from build123d import *

# Parameters (mm, degrees)
SKETCH_2_W          = 180
SKETCH_2_H          = 180
EXTRUDE_1_DEPTH     = 5
EXTRUDE_1_2_DEPTH   = 115
EXTRUDE_2_DEPTH     = 2
CUT_EXTRUDE_1_DEPTH = 140.5
SKETCH_6_R          = 6.5
CUT_EXTRUDE_2_DEPTH = 6
FILLET_1_R          = 10
CUT_EXTRUDE_3_REACH = 141


with BuildPart() as part:
    # Эскиз2 → Extrude 1 (new body)
    with BuildSketch(Plane(origin=(0, 0, 0), x_dir=(1, 0, 0), z_dir=(0, 1, 0))):
        Rectangle(SKETCH_2_W, SKETCH_2_H)
    extrude(amount=EXTRUDE_1_DEPTH)

    # Эскиз3 → Extrude 1 2 (add)
    with BuildSketch(Plane(origin=(0, 5, 0), x_dir=(1, 0, 0), z_dir=(0, 1, 0))):
        with BuildLine():
            Line((-45.5, -45), (-45.5, 44))
            ThreePointArc((-45.5, 44), (-45.207106781, 44.707106781), (-44.5, 45))
            Line((-44.5, 45), (44.5, 45))
            ThreePointArc((44.5, 45), (45.207106781, 44.707106781), (45.5, 44))
            Line((45.5, 44), (45.5, -45))
            Line((45.5, -45), (49.5, -45))
            Line((49.5, -45), (49.5, 44))
            ThreePointArc((49.5, 44), (48.035533906, 47.535533906), (44.5, 49))
            Line((44.5, 49), (-44.5, 49))
            ThreePointArc((-44.5, 49), (-48.035533906, 47.535533906), (-49.5, 44))
            Line((-49.5, 44), (-49.5, -45))
            Line((-49.5, -45), (-45.5, -45))
        make_face()
    extrude(amount=EXTRUDE_1_2_DEPTH)

    # Эскиз4 → Бобышка-Вытянуть2 (add, symmetric)
    with BuildSketch(Plane(origin=(0, 0, 0), x_dir=(0, 0, -1), z_dir=(1, 0, 0))):
        Polygon((49, 67.353829072), (85, 5), (49, 5), align=None)
    extrude(amount=EXTRUDE_2_DEPTH, both=True)

    # Эскиз5 → Вырез-Вытянуть1 (cut, through all)
    with BuildSketch(Plane(origin=(49.5, 0, 0), x_dir=(0, 0, -1), z_dir=(1, 0, 0))):
        with BuildLine():
            Line((-17.5, 108), (-17.5, 96))
            ThreePointArc((-17.5, 96), (-22.5, 91), (-27.5, 96))
            Line((-27.5, 96), (-27.5, 108))
            ThreePointArc((-27.5, 108), (-22.5, 113), (-17.5, 108))
        make_face()
        with BuildLine():
            Line((-17.5, 29), (-17.5, 17))
            ThreePointArc((-17.5, 17), (-22.5, 12), (-27.5, 17))
            Line((-27.5, 17), (-27.5, 29))
            ThreePointArc((-27.5, 29), (-22.5, 34), (-17.5, 29))
        make_face()
        with BuildLine():
            Line((17.5, 108), (17.5, 96))
            ThreePointArc((17.5, 96), (22.5, 91), (27.5, 96))
            Line((27.5, 96), (27.5, 108))
            ThreePointArc((27.5, 108), (22.5, 113), (17.5, 108))
        make_face()
        with BuildLine():
            Line((17.5, 29), (17.5, 17))
            ThreePointArc((17.5, 17), (22.5, 12), (27.5, 17))
            Line((27.5, 17), (27.5, 29))
            ThreePointArc((27.5, 29), (22.5, 34), (17.5, 29))
        make_face()
    extrude(amount=-CUT_EXTRUDE_1_DEPTH, mode=Mode.SUBTRACT)

    # Эскиз6 → Вырез-Вытянуть2 (cut, through all)
    with BuildSketch(Plane(origin=(0, 5, 0), x_dir=(1, 0, 0), z_dir=(0, 1, 0))):
        with Locations(Location((-75, 75, 0), (0, 0, 270))):  # turned: the seam where the file's is
            Circle(SKETCH_6_R)
        with Locations(Location((-75, -75, 0), (0, 0, 270))):  # turned: the seam where the file's is
            Circle(SKETCH_6_R)
        with Locations(Location((75, 75, 0), (0, 0, 270))):  # turned: the seam where the file's is
            Circle(SKETCH_6_R)
        with Locations(Location((75, -75, 0), (0, 0, 270))):  # turned: the seam where the file's is
            Circle(SKETCH_6_R)
    extrude(amount=-CUT_EXTRUDE_2_DEPTH, mode=Mode.SUBTRACT)

    # Скругление1
    fillet_1_edges = [part.edges().sort_by_distance(p)[0] for p in [
        (90, 2.5, 90),
        (-90, 2.5, 90),
        (-90, 2.5, -90),
        (90, 2.5, -90),
    ]]
    fillet(fillet_1_edges, radius=FILLET_1_R)

    # Эскиз8 → Вырез-Вытянуть3 (cut, up to next)
    with BuildSketch(Plane(origin=(0, 0, -49), x_dir=(-1, 0, 0), z_dir=(0, 0, -1)), mode=Mode.PRIVATE) as cut_extrude_3_sk1:
        with BuildLine():
            Line((-17.5, 108), (-17.5, 96))
            ThreePointArc((-17.5, 96), (-22.5, 91), (-27.5, 96))
            Line((-27.5, 96), (-27.5, 108))
            ThreePointArc((-27.5, 108), (-22.5, 113), (-17.5, 108))
        make_face()
    cut_extrude_3_tool1 = extrude(cut_extrude_3_sk1.sketch, amount=-CUT_EXTRUDE_3_REACH, mode=Mode.PRIVATE) & part.part
    add(cut_extrude_3_tool1.solids().sort_by_distance((22.5, 102, -49))[0], mode=Mode.SUBTRACT)
    # Эскиз8 → Вырез-Вытянуть3 (cut, up to next)
    with BuildSketch(Plane(origin=(0, 0, -49), x_dir=(-1, 0, 0), z_dir=(0, 0, -1)), mode=Mode.PRIVATE) as cut_extrude_3_sk2:
        with BuildLine():
            Line((-17.5, 29), (-17.5, 17))
            ThreePointArc((-17.5, 17), (-22.5, 12), (-27.5, 17))
            Line((-27.5, 17), (-27.5, 29))
            ThreePointArc((-27.5, 29), (-22.5, 34), (-17.5, 29))
        make_face()
    cut_extrude_3_tool2 = extrude(cut_extrude_3_sk2.sketch, amount=-CUT_EXTRUDE_3_REACH, mode=Mode.PRIVATE) & part.part
    add(cut_extrude_3_tool2.solids().sort_by_distance((22.5, 23, -49))[0], mode=Mode.SUBTRACT)
    # Эскиз8 → Вырез-Вытянуть3 (cut, up to next)
    with BuildSketch(Plane(origin=(0, 0, -49), x_dir=(-1, 0, 0), z_dir=(0, 0, -1)), mode=Mode.PRIVATE) as cut_extrude_3_sk3:
        with BuildLine():
            Line((17.5, 108), (17.5, 96))
            ThreePointArc((17.5, 96), (22.5, 91), (27.5, 96))
            Line((27.5, 96), (27.5, 108))
            ThreePointArc((27.5, 108), (22.5, 113), (17.5, 108))
        make_face()
    cut_extrude_3_tool3 = extrude(cut_extrude_3_sk3.sketch, amount=-CUT_EXTRUDE_3_REACH, mode=Mode.PRIVATE) & part.part
    add(cut_extrude_3_tool3.solids().sort_by_distance((-22.5, 102, -49))[0], mode=Mode.SUBTRACT)
    # Эскиз8 → Вырез-Вытянуть3 (cut, up to next)
    with BuildSketch(Plane(origin=(0, 0, -49), x_dir=(-1, 0, 0), z_dir=(0, 0, -1)), mode=Mode.PRIVATE) as cut_extrude_3_sk4:
        with BuildLine():
            Line((17.5, 29), (17.5, 17))
            ThreePointArc((17.5, 17), (22.5, 12), (27.5, 17))
            Line((27.5, 17), (27.5, 29))
            ThreePointArc((27.5, 29), (22.5, 34), (17.5, 29))
        make_face()
    cut_extrude_3_tool4 = extrude(cut_extrude_3_sk4.sketch, amount=-CUT_EXTRUDE_3_REACH, mode=Mode.PRIVATE) & part.part
    add(cut_extrude_3_tool4.solids().sort_by_distance((-22.5, 23, -49))[0], mode=Mode.SUBTRACT)


solid = part.part
Read the model definition and answer for the solid it produces. Units are mm, in the model's axes. A direction names the side the tool comes from. Give positions to 0.01 mm unless a question says otherwise; leave off trailing zeros. Write each loop counter-clockwise with the first axis right and the second up, starting at its lowest first coordinate (ties: lowest second). Pieces come first, ordered by that corner, then holes. Notation, with made-up numbers: (77.25, -17.5) - (84.25, -17.5) arc R16 cw to (84.25, 3.5) - close; hole circle Ø5 at (7, 21.5). An arc over 180 degrees is marked (long way). Answer in a Markdown table with one row per item. Add a question column.
Item 1: Section D-D, the plane y = 76.5 is taken. Write down the section's boundary in (x, z), and give its area (3 significant figures).
Item 2: Section B-B, the plane z = 75 is taken. Write down the section's boundary in (x, y), and give its area (3 significant figures).
Item 3: Flat-ended cylindrical pins translate along their axes: P1, Ø2, axis at x = -48, y = 23, coming from the +Z side; P2, Ø8, axis at x = -4, y = 100.5, coming from the +Z side; P3, Ø4.5, axis at y = 22.5, z = -47.5, coming from the -X side. Find the tip coordinate at first contact, or state that the pin passes through.
Item 4: Section C-C, the plane z = -22.5 is taken. Write down the section's boundary in (x, y).
Item 5: Find the intervals of material crossed by L1, parallel to X at y = 3.7, z = -75; L2, parallel to X at y = 81, z = 13; L3, parallel to Y at x = 63, z = -40.5, in increasing order.
Item 6: A tool of negligible diameter and unlimited length cuts with its end or side. For faces 4 (the face through (-9, 62, -49)), 5 (the face through (49.5, 62, 1)), 6 (the face through (-45.5, 62, 1)), from which of +Z, -Z, +X, -X, +Y, -Y can it reach the whole face along a straight path? Write none if from no direction.
Item 7: Determine the mould class of faces 1 (the face through (-87.15, 2.54, 86.99)), 2 (the face through (22.6, 34, -47)), 3 (the face through (47.5, 34, -22.6)) for opening direction X: pulls with the +X half, pulls with the -X half, needs draft (parallel to the pull), parting line crosses it, or undercut.
Item 8: Section A-A, the plane x = 75 is taken. Write down the section's boundary in (y, z), and give its area (3 significant figures).
Recorded:
| question | item | result |
|---|---|---|
| 1 | outline | (-49.5, -44) arc R5 ccw to (-44.5, -49) - (44.5, -49) arc R5 ccw to (49.5, -44) - (49.5, 45) - (45.5, 45) - (45.5, -44) arc R1 cw to (44.5, -45) - (-44.5, -45) arc R1 cw to (-45.5, -44) - (-45.5, 45) - (-49.5, 45) - close |
| 1 | area | 1,110 mm2 |
| 2 | outline | (-90, 0) - (-81.5, 0) - (-81.5, 5) - (-90, 5) - close; (-68.5, 0) - (68.5, 0) - (68.5, 5) - (-68.5, 5) - close; (81.5, 0) - (90, 0) - (90, 5) - (81.5, 5) - close |
| 2 | area | 770 mm2 |
| 3 | P1 | stops at z = 45 |
| 3 | P2 | stops at z = -45 |
| 3 | P3 | stops at x = -49.34 |
| 4 | outline | (-90, 0) - (90, 0) - (90, 5) - (49.5, 5) - (49.5, 12) - (45.5, 12) - (45.5, 5) - (-45.5, 5) - (-45.5, 12) - (-49.5, 12) - (-49.5, 5) - (-90, 5) - close; (-49.5, 34) - (-45.5, 34) - (-45.5, 91) - (-49.5, 91) - close; (-49.5, 113) - (-45.5, 113) - (-45.5, 120) - (-49.5, 120) - close; (45.5, 34) - (49.5, 34) - (49.5, 91) - (45.5, 91) - close; (45.5, 113) - (49.5, 113) - (49.5, 120) - (45.5, 120) - close |
| 5 | L1 | x = -90 to -81.5, -68.5 to 68.5, 81.5 to 90 |
| 5 | L2 | x = -49.5 to -45.5, 45.5 to 49.5 |
| 5 | L3 | y = 0 to 5 |
| 6 | face 4 | -Z, +Y |
| 6 | face 5 | +Z, -Z, +X, +Y |
| 6 | face 6 | +Z, +Y |
| 7 | face 1 | pulls with the -X half |
| 7 | face 2 | undercut |
| 7 | face 3 | needs draft |
| 8 | outline | (0, -90) - (5, -90) - (5, -81.5) - (0, -81.5) - close; (0, -68.5) - (5, -68.5) - (5, 68.5) - (0, 68.5) - close; (0, 81.5) - (5, 81.5) - (5, 90) - (0, 90) - close |
| 8 | area | 770 mm2 |
